For this review, take the finished solid that the model builds, in its own axes (mm). A direction names the side the tool comes from. Coordinates: 2 decimals unless noted, no trailing zeros. Order: outer loops, then holes, each group sorted by start corner. A loop starts at its lowest first (then second) coordinate and runs counter-clockwise, first axis right, second up. Notation, with made-up numbers: (-7, 54.25) -> (47, 54.25) arc R26 cw to (47, 78.25) -> close; hole circle Ø8 at (12, 56). An arc over 180 degrees is marked (long way). Return JSON: item names as keys, results as strings. Group by question number.
Item 1: Take a section at B-B (x = 0.65). Write out the cut boundary in (y, z), then the cut area to 3 significant figures.
Item 2: Take a section at D-D (z = -10.5). Write out the cut boundary in (x, y), then the cut area to 3 significant figures.
Item 3: For line 1 along X through (y, z) = (-2, -50); line 2 along Y through (x, z) = (1, -27.5); line 3 along Z through (x, y) = (0.9, -7.5), list the stretches that pass through material, from the lowest coordinate up.
Item 4: Take a section at A-A (z = -51.5). Write out the cut boundary in (x, y).
Item 5: Take a section at C-C (y = -3). Write out the cut boundary in (x, z).
Item 6: Insertion check: pin 1 (9 mm diameter, centred on y = 1, z = -24.5, fed in from -X); pin 2 (1.6 mm diameter, centred on x = 1.5, z = -22.5, fed in from +Y); pin 3 (3.5 mm diameter, centred on y = 4.85, z = 6.02, fed in from -X); pin 4 (1 mm diameter, centred on x = 1, z = -32.5, fed in from -Y). Each pin has a flat end and moves straight along its axis. Give the tip position at first contact, or say it passes through.
Item 7: Draft analysis for pull direction Z (two halves, no side actions). For faces 4 (the cylindrical face through (0.99, -5.84, 6.49)), 5 (the flat face through (-2, -5, 1)), 6 (the cylindrical face through (0.99, 4.94, 8.02)), state which applies: +Z half, -Z half, draft (parallel to the pull), parting line (faces both ways), or undercut.
Item 8: Machinability: for faces 1 (the flat face through (1, -6, -29)), 2 (the cylindrical face through (-0.03, -9.32, 2.01)), 3 (the cylindrical face through (0.986, 0.216, -48.404)), which of the approach directions +Z, -Z, +X, -X, +Y, -Y give a long, thin tool a straight path to every point of the face, cutting with its end or side? Answer none if there is none.
```python
from build123d import *

# Parameters (mm, degrees)
EXTRUDE_1_DEPTH          = 2
EXTRUDE_START            = -2
SKETCH_1_4_R             = 5
EXTRUDE_2_DEPTH          = 2
CUT_EXTRUDE_1_DEPTH      = 58.563801167
CUT_EXTRUDE_1_DEPTH_BACK = 58.563801167
SKETCH_1_3_R             = 2
FILLET_1_R               = 3


with BuildPart() as part:
    # 草图1 → 凸台-拉伸1 (new body)
    with BuildSketch(Plane(origin=(0, 0, 0), x_dir=(0, 0, -1), z_dir=(1, 0, 0))):
        with BuildLine():
            Line((48.71971979, 0), (0, 0))
            Line((0, 0), (1.157760976, -3.180922138))
            ThreePointArc((1.157760976, -3.180922138), (2.450828184, -4.402761461), (3.234245818, -6))
            Line((3.234245818, -6), (52.183821406, -6))
            ThreePointArc((52.183821406, -6), (48.71971979, -4), (48.71971979, 0))
        make_face()
        with BuildLine():
            Line((1.157760976, -3.180922138), (0, 0))
            Line((0, 0), (-1.236380028, 3.396926208))
            ThreePointArc((-1.236380028, 3.396926208), (-4.311110224, 0.149460393), (-8.753920994, 0.660765061))
            Line((-8.753920994, 0.660765061), (-6.359779991, -5.917083284))
            ThreePointArc((-6.359779991, -5.917083284), (-3.285049794, -2.669617469), (1.157760976, -3.180922138))
        make_face()
        with BuildLine():
            ThreePointArc((56.183821406, -2), (53.219097586, 1.863703305), (48.71971979, 0))
            Line((48.71971979, 0), (52.183821406, 0))
            ThreePointArc((52.183821406, 0), (53.598034968, -0.585786438), (54.183821406, -2))
            ThreePointArc((54.183821406, -2), (53.598034968, -3.414213562), (52.183821406, -4))
            Line((52.183821406, -4), (52.183821406, -6))
            ThreePointArc((52.183821406, -6), (55.01224853, -4.828427125), (56.183821406, -2))
        make_face()
        with BuildLine():
            Line((52.183821406, 0), (48.71971979, 0))
            ThreePointArc((48.71971979, 0), (48.71971979, -4), (52.183821406, -6))
            Line((52.183821406, -6), (52.183821406, -4))
            ThreePointArc((52.183821406, -4), (50.183821406, -2), (52.183821406, 0))
        make_face()
        with BuildLine():
            ThreePointArc((3.234245818, -6), (2.450828184, -4.402761461), (1.157760976, -3.180922138))
            Line((1.157760976, -3.180922138), (2.183821406, -6))
            Line((2.183821406, -6), (3.234245818, -6))
        make_face()
        with BuildLine():
            Line((2.183821406, -6), (1.157760976, -3.180922138))
            ThreePointArc((1.157760976, -3.180922138), (-3.285049794, -2.669617469), (-6.359779991, -5.917083284))
            Line((-6.359779991, -5.917083284), (-5.333719561, -8.736161147))
            Line((-5.333719561, -8.736161147), (-3.454334319, -8.05212086))
            ThreePointArc((-3.454334319, -8.05212086), (-2.258989364, -5.488695332), (0.304436164, -6.684040287))
            Line((0.304436164, -6.684040287), (2.183821406, -6))
        make_face()
        with BuildLine():
            ThreePointArc((-8.753920994, 0.660765061), (-4.311110224, 0.149460393), (-1.236380028, 3.396926208))
            Line((-1.236380028, 3.396926208), (-2.262440458, 6.21600407))
            Line((-2.262440458, 6.21600407), (-4.141825699, 5.531963784))
            ThreePointArc((-4.141825699, 5.531963784), (-4.051595435, 5.195219852), (-4.021210941, 4.847923497))
            ThreePointArc((-4.021210941, 4.847923497), (-5.673914585, 2.878307991), (-7.900596182, 4.16388321))
            Line((-7.900596182, 4.16388321), (-9.779981424, 3.479842924))
            Line((-9.779981424, 3.479842924), (-8.753920994, 0.660765061))
        make_face()
        with BuildLine():
            Line((-2.262440458, 6.21600407), (-1.236380028, 3.396926208))
            ThreePointArc((-1.236380028, 3.396926208), (-1.075295729, 4.114491348), (-1.021210941, 4.847923497))
            ThreePointArc((-1.021210941, 4.847923497), (-8.402014349, 9.244714956), (-8.753920994, 0.660765061))
            Line((-8.753920994, 0.660765061), (-9.779981424, 3.479842924))
            Line((-9.779981424, 3.479842924), (-7.900596182, 4.16388321))
            ThreePointArc((-7.900596182, 4.16388321), (-6.705251227, 6.727308738), (-4.141825699, 5.531963784))
            Line((-4.141825699, 5.531963784), (-2.262440458, 6.21600407))
        make_face()
        with BuildLine():
            ThreePointArc((54.183821406, -2), (53.598034968, -0.585786438), (52.183821406, 0))
            Line((52.183821406, 0), (52.183821406, -4))
            ThreePointArc((52.183821406, -4), (53.598034968, -3.414213562), (54.183821406, -2))
        make_face()
        with BuildLine():
            Line((52.183821406, -4), (52.183821406, 0))
            ThreePointArc((52.183821406, 0), (50.183821406, -2), (52.183821406, -4))
        make_face()
        with BuildLine():
            Line((3.234245818, -6), (2.183821406, -6))
            Line((2.183821406, -6), (0.304436164, -6.684040287))
            ThreePointArc((0.304436164, -6.684040287), (0.394666428, -7.020784218), (0.425050922, -7.368080573))
            ThreePointArc((0.425050922, -7.368080573), (-1.227652722, -9.337696079), (-3.454334319, -8.05212086))
            Line((-3.454334319, -8.05212086), (-5.333719561, -8.736161147))
            Line((-5.333719561, -8.736161147), (-6.359779991, -5.917083284))
            ThreePointArc((-6.359779991, -5.917083284), (-2.308381227, -12.313995785), (3.425050922, -7.368080573))
            ThreePointArc((3.425050922, -7.368080573), (3.377119908, -6.677419469), (3.234245818, -6))
        make_face()
        with BuildLine():
            ThreePointArc((0.425050922, -7.368080573), (0.394666428, -7.020784218), (0.304436164, -6.684040287))
            Line((0.304436164, -6.684040287), (-3.454334319, -8.05212086))
            ThreePointArc((-3.454334319, -8.05212086), (-1.227652722, -9.337696079), (0.425050922, -7.368080573))
        make_face()
        with BuildLine():
            Line((-3.454334319, -8.05212086), (0.304436164, -6.684040287))
            ThreePointArc((0.304436164, -6.684040287), (-2.258989364, -5.488695332), (-3.454334319, -8.05212086))
        make_face()
        with BuildLine():
            ThreePointArc((-4.021210941, 4.847923497), (-4.051595435, 5.195219852), (-4.141825699, 5.531963784))
            Line((-4.141825699, 5.531963784), (-7.900596182, 4.16388321))
            ThreePointArc((-7.900596182, 4.16388321), (-5.673914585, 2.878307991), (-4.021210941, 4.847923497))
        make_face()
        with BuildLine():
            Line((-7.900596182, 4.16388321), (-4.141825699, 5.531963784))
            ThreePointArc((-4.141825699, 5.531963784), (-6.705251227, 6.727308738), (-7.900596182, 4.16388321))
        make_face()
    extrude(amount=EXTRUDE_1_DEPTH)

    # 草图1<4> → 凸台-拉伸2 (add)
    with BuildSketch(Plane(origin=(0, 0, 0), x_dir=(0, 0, -1), z_dir=(1, 0, 0)).offset(EXTRUDE_START)):
        with Locations(Location((-1.574949078, -7.368080573, 0), (0, 0, 163.130102354))):
            Circle(SKETCH_1_4_R)
    extrude(amount=EXTRUDE_2_DEPTH)

    # 草图1<3> → 切除-拉伸1 (cut, two sides: drawn at the far end of the back side and taken through both)
    with BuildSketch(Plane(origin=(0, 0, 0), x_dir=(0, 0, -1), z_dir=(1, 0, 0)).offset(-CUT_EXTRUDE_1_DEPTH_BACK)):
        with Locations((-6.021210941, 4.847923497)):
            Circle(SKETCH_1_3_R)
        with Locations((52.183821406, -2)):
            Circle(SKETCH_1_3_R)
        with Locations((-1.574949078, -7.368080573)):
            Circle(SKETCH_1_3_R)
    extrude(amount=CUT_EXTRUDE_1_DEPTH + CUT_EXTRUDE_1_DEPTH_BACK, mode=Mode.SUBTRACT)

    # 圆角1
    # the kernel refuses this fillet: 3 mm, written as the material it adds along each edge
    with BuildSketch(Plane(origin=(0, -6, -3.234245818), x_dir=(0, 0, -1), z_dir=(1, 0, 0))) as fillet_1_piece_1:
        with BuildLine():
            CenterArc((3.022589, -3), FILLET_1_R, 90, 78.229623191)
            ThreePointArc((0.085670039, -2.388030215), (0.187590709, -1.18882203), (0, 0))
            Line((0, 0), (3.022589, 0))
        make_face()
    extrude(amount=2)
    with BuildSketch(Plane(origin=(0, 0, 0), x_dir=(0, 0, -1), z_dir=(1, 0, 0))) as fillet_1_piece_2:
        with BuildLine():
            CenterArc((FILLET_1_R * 0.70020753821, FILLET_1_R), FILLET_1_R, 200, 70)
            Line((-FILLET_1_R * 0.239485082576, FILLET_1_R * 0.657979856674), (0, 0))
            Line((0, 0), (FILLET_1_R * 0.70020753821, 0))
        make_face()
    extrude(amount=2)
    with BuildSketch(Plane(origin=(0, 0, -48.71971979), x_dir=(0, 0, 1), z_dir=(1, 0, 0))) as fillet_1_piece_3:
        with BuildLine():
            CenterArc((1.43487787, -3), FILLET_1_R, 90, 44.415308597)
            ThreePointArc((-0.664684766, -0.857142857), (-0.303154074, -0.451205957), (0, 0))
            Line((0, 0), (1.43487787, 0))
        make_face()
    extrude(amount=2)
    with BuildSketch(Plane(origin=(0, 0.660765061, 8.753920994), x_dir=(0, 0.6030345104353418, 0.7977150990322344), z_dir=(1, 0, 0))) as fillet_1_piece_4:
        with BuildLine():
            CenterArc((0.897200113, 2.992846785), FILLET_1_R, 237.087538991, 28.955024372)
            Line((-0.732871014, 0.474341649), (0, 0))
            ThreePointArc((0, 0), (0.345076967, 0.011922025), (0.690153933, 0))
        make_face()
    extrude(amount=2)
    with BuildSketch(Plane(origin=(0, -5.917083284, 6.359779991), x_dir=(0, -0.974712617445799, 0.2234621072843435), z_dir=(1, 0, 0))) as fillet_1_piece_5:
        with BuildLine():
            CenterArc((0.897200113, -2.992846785), FILLET_1_R, 93.957436637, 28.955024372)
            Line((-0.732871014, -0.474341649), (0, 0))
            ThreePointArc((0, 0), (0.345076967, -0.011922025), (0.690153933, 0))
        make_face()
    extrude(amount=2)


solid = part.part
```
Findings below:
{
 "1": {"outline": "(-8.39, -3.32) arc R3 cw to (-6, -6.26) -> (-6, -52.18) arc R4 ccw (long way) to (0.86, -49.38) arc R3 cw to (0, -47.28) -> (0, -2.1) arc R3 cw to (1.97, 0.72) -> (3.4, 1.24) arc R5 ccw (long way) to (1.08, 9.3) arc R3 cw to (-0.16, 8.46) -> (-5.1, 6.66) arc R3 cw to (-6.59, 6.51) arc R5 ccw to start; hole circle Ø4 at (-7.37, 1.57); hole circle Ø4 at (-2, -52.18); hole circle Ø4 at (4.85, 6.02)", "area": "490 mm2"},
 "2": {"outline": "(0, -6) -> (2, -6) -> (2, 0) -> (0, 0) -> close", "area": "12.0 mm2"},
 "3": {"line 1": "x = 0 to 2", "line 2": "y = -6 to 0", "line 3": "z = -3.66 to -0.42, 3.57 to 6.57"},
 "4": {"outline": "(0, -6) -> (2, -6) -> (2, -3.88) -> (0, -3.88) -> close; (0, -0.12) -> (2, -0.12) -> (2, 1.94) -> (0, 1.94) -> close"},
 "5": {"outline": "(-2, -0.86) -> (0, -0.86) -> (0, -50.45) -> (2, -50.45) -> (2, 7.42) -> (0, 7.42) -> (0, 4.01) -> (-2, 4.01) -> close; (0, -56.06) -> (2, -56.06) -> (2, -53.92) -> (0, -53.92) -> close"},
 "6": {"pin 1": "stops at x = 0", "pin 2": "stops at y = 0", "pin 3": "passes through", "pin 4": "stops at y = -6"},
 "7": {"face 4": "+Z half", "face 5": "draft", "face 6": "undercut"},
 "8": {"face 1": "-Z, +X, -X, -Y", "face 2": "+X, -X", "face 3": "+X, -X, +Y"}
}
